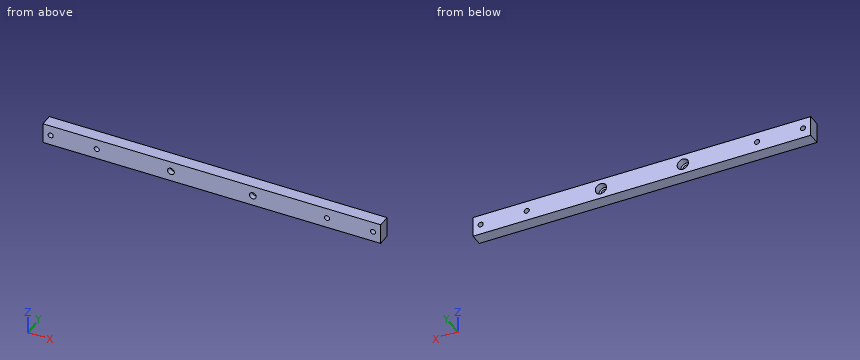
from build123d import *

# Parameters (mm, degrees)
SKETCH_1_W                = 330
SKETCH_1_H                = 20
EXTRUDE_1_DEPTH           = 12
HOLE_WIZARD_M6_1_D        = 5
HOLE_WIZARD_M6_1_DEPTH    = 15
HOLE_WIZARD_M6_1_TIP      = 1.502151548
HOLE_WIZARD_1_D           = 6.6
HOLE_WIZARD_1_CBORE_D     = 11
HOLE_WIZARD_1_CBORE_DEPTH = 6.8


with BuildPart() as part:
    # 草图1 → 凸台-拉伸1 (new body)
    with BuildSketch(Plane(origin=(0, 0, 0), x_dir=(1, 0, 0), z_dir=(0, 1, 0))):
        Rectangle(SKETCH_1_W, SKETCH_1_H)
    extrude(amount=EXTRUDE_1_DEPTH)

    # M6 螺纹孔1
    with Locations(Plane(origin=(0, 12, 0), x_dir=(1, 0, 0), z_dir=(0, 1, 0))):
        with Locations((-157.5, 0), (-112.5, 0), (112.5, 0), (157.5, 0)):
            Hole(HOLE_WIZARD_M6_1_D / 2, depth=HOLE_WIZARD_M6_1_DEPTH)
            with Locations((0, 0, -(HOLE_WIZARD_M6_1_DEPTH + HOLE_WIZARD_M6_1_TIP / 2))):  # 118° drill point
                Cone(0, HOLE_WIZARD_M6_1_D / 2, HOLE_WIZARD_M6_1_TIP, mode=Mode.SUBTRACT)

    # 打孔尺寸根据内六角圆柱头螺钉的类型1 (through all)
    with Locations(Plane(origin=(0, 12, 0), x_dir=(1, 0, 0), z_dir=(0, 1, 0))):
        with Locations((-40, 0), (40, 0)):
            CounterBoreHole(HOLE_WIZARD_1_D / 2, HOLE_WIZARD_1_CBORE_D / 2, HOLE_WIZARD_1_CBORE_DEPTH)


solid = part.part
Could you check a few things on this model? Use its own coordinates, in mm. Give positions to 0.01 mm unless a question says otherwise; leave off trailing zeros. Order: outer loops, then holes, each group sorted by start corner. A loop starts at its lowest first (then second) coordinate and runs counter-clockwise, first axis right, second up.
1. Suppose I cut it at B-B (y = 8). List the corners of the cut face in (x, z) for me.
2. I need wall thicknesses on L1, parallel to Z at x = 40, y = 2.25; L2, parallel to Z at x = -40, y = 8.5; L3, parallel to X at y = 10, z = -3.5. Which ranges of each line are inside material? Lowest first, please.
3. Suppose I cut it at A-A (x = -40). List the corners of the cut face in (y, z) for me, plus the area to 3 significant figures.
4. Will these pins go through, and if not, where does the flat tip stop? P1, Ø6.5, axis at x = 112.5, z = 0, coming from the +Y side; P2, Ø3.5, axis at x = -41.5, z = 0.5, coming from the +Y side; P3, Ø3, axis at x = -157.5, z = 0, coming from the -Y side.
Solved:
1. outline: (-165, -10) - (165, -10) - (165, 10) - (-165, 10) - close; hole circle Ø5 at (-157.5, 0); hole circle Ø5 at (-112.5, 0); hole circle Ø11 at (-40, 0); hole circle Ø11 at (40, 0); hole circle Ø5 at (112.5, 0); hole circle Ø5 at (157.5, 0)
2. L1: z = -10 to -3.3, 3.3 to 10
2. L2: z = -10 to -5.5, 5.5 to 10
2. L3: x = -165 to -44.24, -35.76 to 35.76, 44.24 to 165
3. outline: (0, -10) - (12, -10) - (12, -5.5) - (5.2, -5.5) - (5.2, -3.3) - (0, -3.3) - close; (0, 3.3) - (5.2, 3.3) - (5.2, 5.5) - (12, 5.5) - (12, 10) - (0, 10) - close
3. area: 131 mm2
4. P1: stops at y = 12
4. P2: stops at y = 5.2
4. P3: passes through
